Could you check a few things on this model? Use its own coordinates, in mm. Coordinates: 2 decimals unless noted, no trailing zeros. Order: outer loops, then holes, each group sorted by start corner. A loop starts at its lowest first (then second) coordinate and runs counter-clockwise, first axis right, second up. Notation, with made-up numbers: (57, 5.5) - (84, 5.5) arc R30 ccw to (84, 41.5) - close; hole circle Ø10 at (44, -36). An arc over 180 degrees is marked (long way). Answer as CSV lines item,"result". Start each with the question number.
1. I want a section at B-B, the plane x = 188. List the corners of the cut face in (y, z) for me (3 decimals).
2. I need wall thicknesses on probe 1 along Z at (x, y) = (1060, 4.5) (3 decimals); probe 2 along Z at (x, y) = (1053, 1.5) (3 decimals); probe 3 along Y at (x, z) = (419, -11.25) (3 decimals). Which ranges of each line are inside material? Lowest first, please.
3. I want a section at A-A, the plane y = 4.25. List the corners of the cut face in (x, z) for me (3 decimals), and give its area (3 significant figures).
4. For pin 1 (3.5 mm diameter, centred on x = 1193.8, z = -7.94, fed in from -Y), with a flat end and sliding along its axis, tell me the tip position at first contact or that it passes through.
from build123d import *

# Parameters (mm, degrees)
SKETCH1_W           = 15.875
SKETCH1_H           = 15.875
BOSS_EXTRUDE1_DEPTH = 1219.2
SKETCH2_R           = 2
CUT_EXTRUDE1_DEPTH  = 16.875


with BuildPart() as part:
    # Sketch1 → Boss-Extrude1 (new body)
    with BuildSketch(Plane(origin=(0, 0, 0), x_dir=(0, 0, -1), z_dir=(1, 0, 0))):
        with Locations((7.9375, 7.9375)):
            Rectangle(SKETCH1_W, SKETCH1_H)
        with BuildLine():
            Line((1.7446, 1.2446), (14.1304, 1.2446))
            ThreePointArc((14.1304, 1.2446), (14.483953391, 1.391046609), (14.6304, 1.7446))
            Line((14.6304, 1.7446), (14.6304, 14.1304))
            ThreePointArc((14.6304, 14.1304), (14.483953391, 14.483953391), (14.1304, 14.6304))
            Line((14.1304, 14.6304), (1.7446, 14.6304))
            ThreePointArc((1.7446, 14.6304), (1.391046609, 14.483953391), (1.2446, 14.1304))
            Line((1.2446, 14.1304), (1.2446, 1.7446))
            ThreePointArc((1.2446, 1.7446), (1.391046609, 1.391046609), (1.7446, 1.2446))
        make_face(mode=Mode.SUBTRACT)
    extrude(amount=BOSS_EXTRUDE1_DEPTH)

    # Sketch2 → Cut-Extrude1 (cut, through all)
    with BuildSketch(Plane(origin=(0, 15.875, 0), x_dir=(1, 0, 0), z_dir=(0, 1, 0))):
        with Locations((609.600483099, 6.875)):
            Circle(SKETCH2_R)
        with Locations((25.4, 6.875)):
            Circle(SKETCH2_R)
        with Locations((1193.8, 7.9375)):
            Circle(SKETCH2_R)
    extrude(amount=-CUT_EXTRUDE1_DEPTH, mode=Mode.SUBTRACT)


solid = part.part
Solved:
1,outline,"(0, -15.875) - (15.875, -15.875) - (15.875, 0) - (0, 0) - close; hole (1.245, -14.13) arc R0.5 ccw to (1.745, -14.63) - (14.13, -14.63) arc R0.5 ccw to (14.63, -14.13) - (14.63, -1.745) arc R0.5 ccw to (14.13, -1.245) - (1.745, -1.245) arc R0.5 ccw to (1.245, -1.745) - close"
2,probe 1,"z = -15.875 to -14.63, -1.245 to 0"
2,probe 2,"z = -15.875 to -14.566, -1.309 to 0"
2,probe 3,"y = 0 to 1.245, 14.63 to 15.875"
3,outline,"(0, -15.875) - (1219.2, -15.875) - (1219.2, -14.63) - (0, -14.63) - close; (0, -1.245) - (1219.2, -1.245) - (1219.2, 0) - (0, 0) - close"
3,area,"3,030 mm2"
4,pin 1,"passes through"
